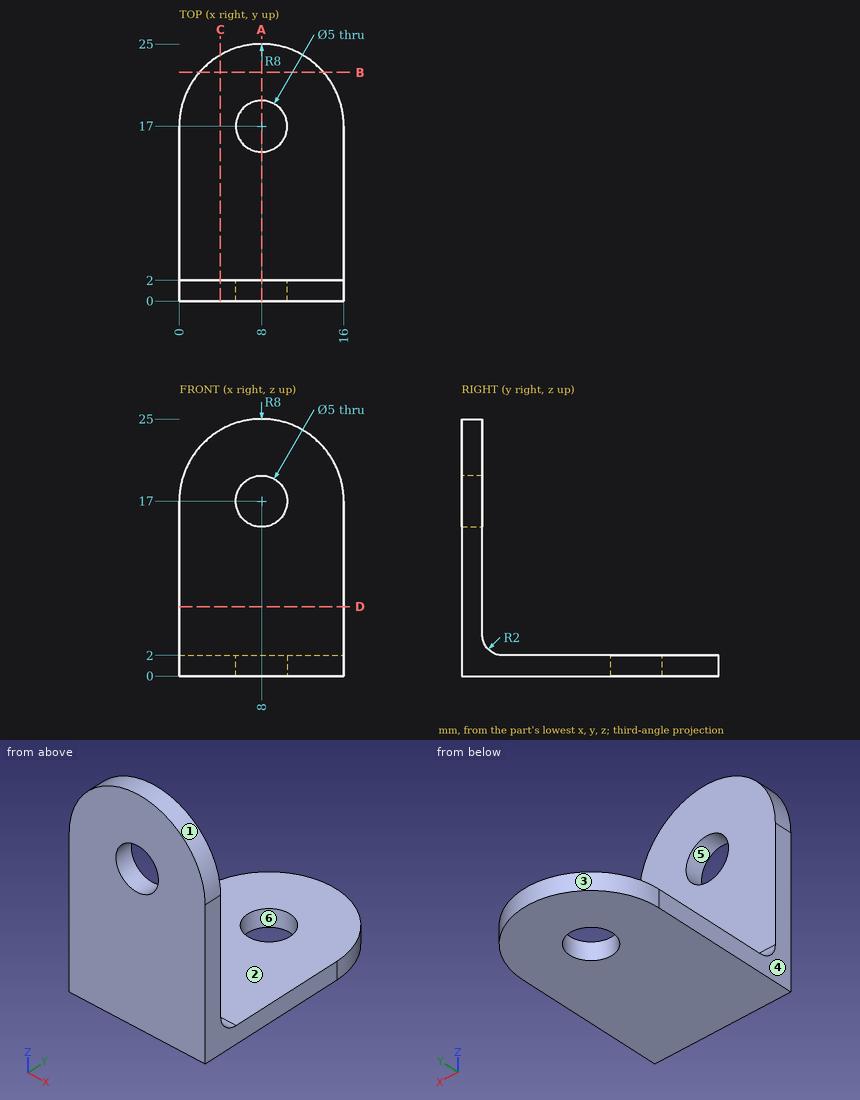
Answer from the drawing. Dimensions are ordinates in mm from the lowest x, y and z of the part. A direction names the side the tool comes from. Give positions to 0.01 mm unless a question says otherwise; leave off trailing zeros. Loops run counter-clockwise (first coordinate to the right, second up) from the corner with the lowest first, then second, coordinate; pieces in that order, holes last. Notation, with made-up numbers: (70.5, 43.5) -> (78.5, 43.5) arc R21 ccw to (78.5, 76.5) -> close; hole circle Ø7 at (59, 39). An arc over 180 degrees is marked (long way). Use a Markdown table: item, result.
Q1. Determine the mould class of the marked faces 3, 4, 5 and 6 for opening direction X: pulls with the +X half, pulls with the -X half, needs draft (parallel to the pull), parting line crosses it, or undercut.
Solved:
| item | result |
|---|---|
| face 3 | parting line crosses it |
| face 4 | pulls with the -X half |
| face 5 | undercut |
| face 6 | undercut |
Q2. Section C-C, the plane x = 4 is taken. Determine the outline of the cut face in (y, z), then the cut area to 3 significant figures.
Solved:
| item | result |
|---|---|
| outline | (0, 0) -> (23.93, 0) -> (23.93, 2) -> (4, 2) arc R2 cw to (2, 4) -> (2, 23.93) -> (0, 23.93) -> close |
| area | 92.6 mm^2 |
Q3. Find the intervals of material crossed by line 1 along X through (y, z) = (1.2, 17); line 2 along Y through (x, z) = (8, 0.45); line 3 along Z through (x, y) = (4.25, 11.5), in increasing order.
Solved:
| item | result |
|---|---|
| line 1 | x = 0 to 5.5, 10.5 to 16 |
| line 2 | y = 0 to 14.5, 19.5 to 25 |
| line 3 | z = 0 to 2 |
Q4. A tool of negligible diameter and unlimited length cuts with its end or side. For the marked faces 1 and 2, from which of +Z, -Z, +X, -X, +Y, -Y can it reach the whole face along a straight path? Write none if from no direction.
Solved:
| item | result |
|---|---|
| face 1 | +Z, +Y, -Y |
| face 2 | +Z, +X, -X, +Y |
Q5. Section D-D, the plane z = 6.75 is taken. Determine the outline of the cut face in (x, y), then the cut area to 3 significant figures.
Solved:
| item | result |
|---|---|
| outline | (0, 0) -> (16, 0) -> (16, 2) -> (0, 2) -> close |
| area | 32.0 mm^2 |
Q6. Section A-A, the plane x = 8 is taken. Determine the outline of the cut face in (y, z), then the cut area to 3 significant figures.
Solved:
| item | result |
|---|---|
| outline | (0, 0) -> (14.5, 0) -> (14.5, 2) -> (4, 2) arc R2 cw to (2, 4) -> (2, 14.5) -> (0, 14.5) -> close; (0, 19.5) -> (2, 19.5) -> (2, 25) -> (0, 25) -> close; (19.5, 0) -> (25, 0) -> (25, 2) -> (19.5, 2) -> close |
| area | 76.9 mm^2 |
Q7. Section B-B, the plane y = 22.25 is taken. Determine the outline of the cut face in (x, z), then the cut area to 3 significant figures.
Solved:
| item | result |
|---|---|
| outline | (1.96, 0) -> (14.04, 0) -> (14.04, 2) -> (1.96, 2) -> close |
| area | 24.1 mm^2 |
Q8. Each of these flat-tipped pins is pushed along its axis until it touches: pin 1 (6 mm diameter, centred on x = 8, z = 17, fed in from +Y); pin 2 (2 mm diameter, centred on y = 4.5, z = 14.5, fed in from -X). Where does it stop, or does it pass through?
Solved:
| item | result |
|---|---|
| pin 1 | stops at y = 2 |
| pin 2 | passes through |
